Source: CAD feature listing. Evaluate the final solid. Frame: model axes, mm. A direction names the side the tool comes from. Give positions to 0.01 mm unless a question says otherwise; leave off trailing zeros. Loops run counter-clockwise (first coordinate to the right, second up) from the corner with the lowest first, then second, coordinate; pieces in that order, holes last. Notation, with made-up numbers: M 29.5,-34.5 L 76.5,-34.5 A14 cw 76.5,-18.5 Z; hole C 22,-19.75 d6. An arc over 180 degrees is marked long. Write item = value, one per line.
from build123d import *

# Parameters (mm, degrees)
F0_R      = 24.5
F0_R_2    = 15
F1_DEPTH  = 2
F2_R      = 15
F3_DEPTH  = 14
F5_DEPTH  = 11.2
F6_R      = 10
F6_R_2    = 9
F7_DEPTH  = 14
F8_DEPTH  = 25
F10_D     = 4.4
F11_SIZE2 = 0.49999
F11_SIZE  = 0.49999


# Not quite as in the source:
# - a fillet or chamfer is up to 0.001 mm smaller than in the source, because OpenCascade refuses the exact size


with BuildPart() as f1:
    # F0 (on Top) → F1 (new body)
    with BuildSketch(Plane.XY):
        Circle(F0_R)
        Circle(F0_R_2, mode=Mode.SUBTRACT)
    extrude(amount=F1_DEPTH)

    # F2 (on Top) → F3 (join)
    with BuildSketch(Plane.XY):
        Circle(F2_R)
    extrude(amount=F3_DEPTH)

    # F4 (on face) → F5 (cut)
    with BuildSketch(Plane.XY.offset(14)):
        with BuildLine():
            ThreePointArc((7.4375, -2.9467938085), (7.8581168228, -1.5), (8, 0))
            ThreePointArc((8, 0), (7.8581168228, 1.5), (7.4375, 2.9467938085))
            ThreePointArc((7.4375, 2.9467938085), (5.6568542495, 5.6568542495), (2.9467938085, 7.4375))
            ThreePointArc((2.9467938085, 7.4375), (0, 8), (-2.9467938085, 7.4375))
            ThreePointArc((-2.9467938085, 7.4375), (-5.6568542495, 5.6568542495), (-7.4375, 2.9467938085))
            ThreePointArc((-7.4375, 2.9467938085), (-8, 0), (-7.4375, -2.9467938085))
            ThreePointArc((-7.4375, -2.9467938085), (-5.6568542495, -5.6568542495), (-2.9467938085, -7.4375))
            ThreePointArc((-2.9467938085, -7.4375), (0, -8), (2.9467938085, -7.4375))
            ThreePointArc((2.9467938085, -7.4375), (5.6568542495, -5.6568542495), (7.4375, -2.9467938085))
        make_face()
        with BuildLine():
            ThreePointArc((7.4375, 2.9467938085), (7.8581168228, 1.5), (8, 0))
            ThreePointArc((8, 0), (7.8581168228, -1.5), (7.4375, -2.9467938085))
            ThreePointArc((7.4375, -2.9467938085), (11, 0), (7.4375, 2.9467938085))
        make_face()
        with BuildLine():
            ThreePointArc((-2.9467938085, 7.4375), (0, 8), (2.9467938085, 7.4375))
            ThreePointArc((2.9467938085, 7.4375), (0, 11), (-2.9467938085, 7.4375))
        make_face()
        with BuildLine():
            ThreePointArc((-2.9467938085, -7.4375), (0, -11), (2.9467938085, -7.4375))
            ThreePointArc((2.9467938085, -7.4375), (0, -8), (-2.9467938085, -7.4375))
        make_face()
        with BuildLine():
            ThreePointArc((-7.4375, -2.9467938085), (-8, 0), (-7.4375, 2.9467938085))
            ThreePointArc((-7.4375, 2.9467938085), (-11, 0), (-7.4375, -2.9467938085))
        make_face()
    extrude(amount=-F5_DEPTH, mode=Mode.SUBTRACT)

    # F6 (on face) → F7 (join)
    with BuildSketch(Plane.XY.offset(2.8)):
        Circle(F6_R)
        Circle(F6_R_2, mode=Mode.SUBTRACT)
    extrude(amount=-F7_DEPTH)

    # F8 (cut): a face of the model
    f8_faces = [f1.faces().sort_by_distance(p)[0] for p in [
        (0, 0, 0),
    ]]
    extrude(f8_faces, amount=-F8_DEPTH, mode=Mode.SUBTRACT)

    # F10 (through all)
    with Locations(Plane.XY.offset(2)):
        with Locations((0, 17.375), (-15.0471913908, -8.6875), (15.0471913908, -8.6875)):
            Hole(F10_D / 2)

    # F11 (size 0.5 and 0.5 in the source; OpenCascade refuses exactly that, so slightly less here)
    f11_edges = [f1.edges().sort_by_distance(p)[0] for p in [
        (-15, 0, 14),
        (-24.5, 0, 2),
        (-24.5, 0, 0),
        (0, 11, 14),
        (11, 0, 14),
        (0, -11, 14),
        (-11, 0, 14),
        (-10, 0, -11.2),
        (-9, 0, -11.2),
    ]]
    chamfer(f11_edges, length=F11_SIZE, length2=F11_SIZE2)


solid = f1.part
1. Reachability of faces 1 (the flat face through (10.3, 0.3, 0)), 2 (the cylindrical face through (12.949, -8.027, 0.986)), 3 (the cylindrical face through (11, 0, 8)) from +Z, -Z, +X, -X, +Y, -Y: full face, straight path, thin tool, end or side. Return the list, or none.
Derived:
face_1 = -Z
face_2 = +Z, -Z
face_3 = +Z
2. Pull-direction query (X, two-part tool) for faces 4 (the flat face through (16, 0, 2)), 5 (the cylindrical face through (-2.17, -9.76, -5.28)), 6 (the flat face through (10, 0, 2.8)); classes: +X half, -X half, draft (parallel to the pull), parting line (faces both ways), or undercut.
Derived:
face_4 = draft
face_5 = parting line
face_6 = undercut
3. First-contact query: pin 1 Ø2 at (y, z) = (7, 5) entering from -X; pin 2 Ø12 at (x, z) = (0.5, -7) entering from +Y; pin 3 Ø1.5 at (x, y) = (-13, -12) entering from -Z. Flat tips, straight axial feed; report the tip coordinate or a pass-through.
Derived:
pin_1 = -13.75
pin_2 = 10
pin_3 = 0
4. Cut plane A-A, the plane z = 10.25. Return the cut outline in (x, y).
Derived:
outline = C 0,0 d30; hole M -8.5,-2.96 A9 ccw -2.96,-8.5 A3 ccw 2.96,-8.5 A9 ccw 8.5,-2.96 A3 ccw 8.5,2.96 A9 ccw 2.96,8.5 A3 ccw -2.96,8.5 A9 ccw -8.5,2.96 A3 ccw Z
5. Material intervals for probe 1 along Y at (x, z) = (0, 1.55) (3 decimals); probe 2 along Z at (x, y) = (-4.5, -17); probe 3 along Z at (x, y) = (3.5, -10.5), sorted ascending. Write a range as from..to.
Derived:
probe_1 = -24.45..-9, 9..15.175, 19.575..24.45
probe_2 = 0..2
probe_3 = 0..14
6. Cut plane C-C, the plane x = 0. Count the separate pieces of the cut face and the enclosed holes in it, then the cut area to 3 significant figures.
Derived:
separate_pieces = 3
enclosed_holes = 0
area = 173 mm²
